from build123d import *

# Parameters (mm, degrees)
F0_R     = 4.6
F0_R_2   = 2.25
F1_DEPTH = 3


with BuildPart() as f1:
    # F0 (on Top) → F1 (new body)
    with BuildSketch(Plane.XY):
        with BuildLine():
            ThreePointArc((40.45085, 29.389263), (29.389263, 40.45085), (15.45085, 47.552826))
            ThreePointArc((15.45085, 47.552826), (0, 50), (-15.45085, 47.552826))
            ThreePointArc((-15.45085, 47.552826), (-29.389263, 40.45085), (-40.45085, 29.389263))
            ThreePointArc((-40.45085, 29.389263), (-47.552826, 15.45085), (-50, 0))
            ThreePointArc((-50, 0), (-47.552826, -15.45085), (-40.45085, -29.389263))
            ThreePointArc((-40.45085, -29.389263), (-29.389263, -40.45085), (-15.45085, -47.552826))
            ThreePointArc((-15.45085, -47.552826), (0, -50), (15.45085, -47.552826))
            ThreePointArc((15.45085, -47.552826), (29.389263, -40.45085), (40.45085, -29.389263))
            ThreePointArc((40.45085, -29.389263), (47.552826, -15.45085), (50, 0))
            ThreePointArc((50, 0), (47.552826, 15.45085), (40.45085, 29.389263))
        make_face()
        with Locations((-20.572484, -28.315595)):
            Circle(F0_R, mode=Mode.SUBTRACT)
        with Locations((-33.286978, -10.815595)):
            Circle(F0_R, mode=Mode.SUBTRACT)
        with Locations((-13.468813, -18.538231)):
            Circle(F0_R_2, mode=Mode.SUBTRACT)
        with Locations((-21.792998, -7.080974)):
            Circle(F0_R_2, mode=Mode.SUBTRACT)
        with Locations((0, -35)):
            Circle(F0_R, mode=Mode.SUBTRACT)
        with Locations((20.572484, -28.315595)):
            Circle(F0_R, mode=Mode.SUBTRACT)
        with Locations((0, -22.914514)):
            Circle(F0_R_2, mode=Mode.SUBTRACT)
        with Locations((13.468813, -18.538231)):
            Circle(F0_R_2, mode=Mode.SUBTRACT)
        with BuildLine():
            ThreePointArc((-3.399187, 10.461622), (0, 11), (3.399187, 10.461622))
            ThreePointArc((3.399187, 10.461622), (6.465638, 8.899187), (8.899187, 6.465638))
            ThreePointArc((8.899187, 6.465638), (10.461622, 3.399187), (11, 0))
            ThreePointArc((11, 0), (10.461622, -3.399187), (8.899187, -6.465638))
            ThreePointArc((8.899187, -6.465638), (6.465638, -8.899187), (3.399187, -10.461622))
            ThreePointArc((3.399187, -10.461622), (0, -11), (-3.399187, -10.461622))
            ThreePointArc((-3.399187, -10.461622), (-6.465638, -8.899187), (-8.899187, -6.465638))
            ThreePointArc((-8.899187, -6.465638), (-10.461622, -3.399187), (-11, 0))
            ThreePointArc((-11, 0), (-10.461622, 3.399187), (-8.899187, 6.465638))
            ThreePointArc((-8.899187, 6.465638), (-6.465638, 8.899187), (-3.399187, 10.461622))
        make_face(mode=Mode.SUBTRACT)
        with Locations((21.792998, -7.080974)):
            Circle(F0_R_2, mode=Mode.SUBTRACT)
        with Locations((33.286978, -10.815595)):
            Circle(F0_R, mode=Mode.SUBTRACT)
        with Locations((-33.286978, 10.815595)):
            Circle(F0_R, mode=Mode.SUBTRACT)
        with Locations((-21.792998, 7.080974)):
            Circle(F0_R_2, mode=Mode.SUBTRACT)
        with Locations((-13.468813, 18.538231)):
            Circle(F0_R_2, mode=Mode.SUBTRACT)
        with Locations((-20.572484, 28.315595)):
            Circle(F0_R, mode=Mode.SUBTRACT)
        with Locations((21.792998, 7.080974)):
            Circle(F0_R_2, mode=Mode.SUBTRACT)
        with Locations((0, 22.914514)):
            Circle(F0_R_2, mode=Mode.SUBTRACT)
        with Locations((13.468813, 18.538231)):
            Circle(F0_R_2, mode=Mode.SUBTRACT)
        with Locations((33.286978, 10.815595)):
            Circle(F0_R, mode=Mode.SUBTRACT)
        with Locations((0, 35)):
            Circle(F0_R, mode=Mode.SUBTRACT)
        with Locations((20.572484, 28.315595)):
            Circle(F0_R, mode=Mode.SUBTRACT)
    extrude(amount=F1_DEPTH)


solid = f1.part
Input: part model. Units: mm. Frame: model coordinates. Give positions to 0.01 mm unless a question says otherwise; leave off trailing zeros. Loops run counter-clockwise (first coordinate to the right, second up) from the corner with the lowest first, then second, coordinate; pieces in that order, holes last. Notation, with made-up numbers: (37.5, 78) - (81.5, 78) arc R7 cw to (81.5, 88) - close; hole circle Ø10 at (-0.75, -9). An arc over 180 degrees is marked (long way). Use CSV: the item, a comma, the result in double quotes. Start each with the question number.
Item 1: Section D-D on y = -35. Return loops of the section in (x, z), then the cut area to 3 significant figures.
Item 2: Contact query for a flat-ended pin moving along its axis: P1, Ø1, axis at y = -8, z = 1.5, coming from the -X side. Output: stop coordinate, or through.
Item 3: Section B-B on x = -33. Return loops of the section in (y, z).
Item 4: Section A-A on x = 0. Return loops of the section in (y, z).
Item 5: Mould query, pull axis X, two halves, no side actions, for faces 1 (the cylindrical face through (14.507, 16.542, 1.479)), 2 (the flat face through (-1, 12, 3)). Classes: pulls with the +X half, pulls with the -X half, needs draft (parallel to the pull), parting line crosses it, or undercut.
Item 6: Section C-C on y = 14. Return loops of the section in (x, z).
Item 7: Line query: line 1 (Y direction, x = 0, z = 2.1); line 2 (X direction, y = -30, z = 0.6); line 3 (X direction, y = 7.5, z = 2). Output: solid intervals per line, ascending.
Ans:
1,outline,"(-35.71, 0) - (-4.6, 0) - (-4.6, 3) - (-35.71, 3) - close; (4.6, 0) - (35.71, 0) - (35.71, 3) - (4.6, 3) - close"
1,area,"187 mm2"
2,P1,"stops at x = -49.43"
3,outline,"(-37.56, 0) - (-15.41, 0) - (-15.41, 3) - (-37.56, 3) - close; (-6.22, 0) - (6.22, 0) - (6.22, 3) - (-6.22, 3) - close; (15.41, 0) - (37.56, 0) - (37.56, 3) - (15.41, 3) - close"
4,outline,"(-50, 0) - (-39.6, 0) - (-39.6, 3) - (-50, 3) - close; (-30.4, 0) - (-25.16, 0) - (-25.16, 3) - (-30.4, 3) - close; (-20.66, 0) - (-11, 0) - (-11, 3) - (-20.66, 3) - close; (11, 0) - (20.66, 0) - (20.66, 3) - (11, 3) - close; (25.16, 0) - (30.4, 0) - (30.4, 3) - (25.16, 3) - close; (39.6, 0) - (50, 0) - (50, 3) - (39.6, 3) - close"
5,face 1,"undercut"
5,face 2,"needs draft"
6,outline,"(-48, 0) - (-36.61, 0) - (-36.61, 3) - (-48, 3) - close; (-29.97, 0) - (29.97, 0) - (29.97, 3) - (-29.97, 3) - close; (36.61, 0) - (48, 0) - (48, 3) - (36.61, 3) - close"
7,line 1,"y = -50 to -39.6, -30.4 to -25.16, -20.66 to -11, 11 to 20.66, 25.16 to 30.4, 39.6 to 50"
7,line 2,"x = -40 to -24.85, -16.29 to 16.29, 24.85 to 40"
7,line 3,"x = -49.43 to -36.48, -30.1 to -24, -19.58 to -8.05, 8.05 to 19.58, 24 to 30.1, 36.48 to 49.43"
